Design review of the part shown in the three views and the two pictorial views. Dimensions are in mm from the part's minimum x, y and z. Round coordinates to 2 decimals unless told otherwise and drop trailing zeros. Write each loop counter-clockwise with the first axis right and the second up, starting at its lowest first coordinate (ties: lowest second). Pieces come first, ordered by that corner, then holes. Notation, with made-up numbers: (27.5, 36.5) -> (69.5, 36.5) arc R33 ccw to (69.5, 66.5) -> close; hole circle Ø8 at (-1, -34). An arc over 180 degrees is marked (long way). Return JSON: item names as keys, results as strings. Group by question number.
1. Take a section at B-B, the plane y = 114.3. Write out the cut boundary in (x, z) (1 decimal).
2. For line 1 along Y through (x, z) = (38.1, 1.3); line 2 along X through (y, z) = (116, 3); line 3 along Y through (x, z) = (34.5, 0.25) (1 decimal), list the stretches that pass through material, from the lowest coordinate up. Write a range as from..to.
3. Take a section at D-D, the plane x = 38.1. Write out the cut boundary in (y, z) (1 decimal).
4. Take a section at A-A, the plane z = 2.2. Write out the cut boundary in (x, y).
5. Clearance check with a flat-ended pin moving along its axis: P1, Ø16, axis at x = 38.1, y = 190.5, coming from the -Z side. State where the tip first meets the part, or that it passes through.
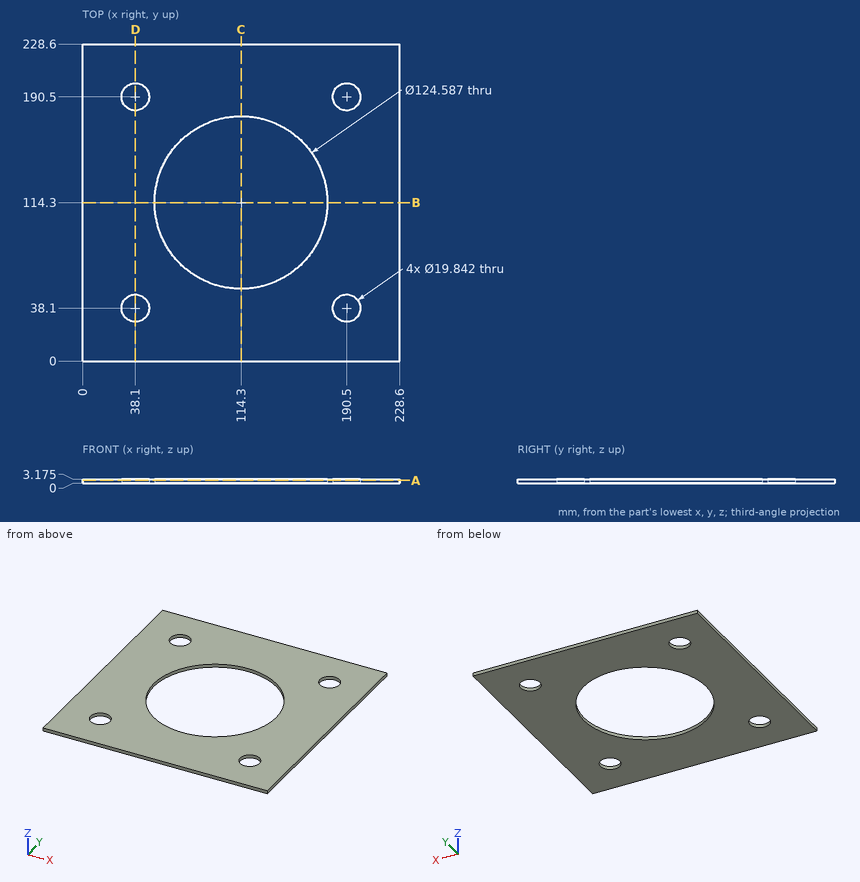
Output:
{
 "1": {"outline": "(0, 0) -> (52, 0) -> (52, 3.2) -> (0, 3.2) -> close; (176.6, 0) -> (228.6, 0) -> (228.6, 3.2) -> (176.6, 3.2) -> close"},
 "2": {"line 1": "y = 0..28.18, 48.02..180.58, 200.42..228.6", "line 2": "x = 0..52.03, 176.57..228.6", "line 3": "y = 0..28.9, 47.3..181.3, 199.7..228.6"},
 "3": {"outline": "(0, 0) -> (28.2, 0) -> (28.2, 3.2) -> (0, 3.2) -> close; (48, 0) -> (180.6, 0) -> (180.6, 3.2) -> (48, 3.2) -> close; (200.4, 0) -> (228.6, 0) -> (228.6, 3.2) -> (200.4, 3.2) -> close"},
 "4": {"outline": "(0, 0) -> (228.6, 0) -> (228.6, 228.6) -> (0, 228.6) -> close; hole circle Ø19.84 at (38.1, 38.1); hole circle Ø19.84 at (38.1, 190.5); hole circle Ø124.59 at (114.3, 114.3); hole circle Ø19.84 at (190.5, 38.1); hole circle Ø19.84 at (190.5, 190.5)"},
 "5": {"P1": "passes through"}
}
